Check sheet for the modelled part. Datum: model origin and axes. Units: mm. A direction names the side the tool comes from. Give positions to 0.01 mm unless a question says otherwise; leave off trailing zeros. Order: outer loops, then holes, each group sorted by start corner. A loop starts at its lowest first (then second) coordinate and runs counter-clockwise, first axis right, second up.
```python
from build123d import *

# Parameters (mm, degrees)
SKETCH1_W                = 30
SKETCH1_H                = 115
BOSS_EXTRUDE1_DEPTH      = 6.5
BOSS_EXTRUDE2_DEPTH      = 21.025
BOSS_EXTRUDE2_DEPTH_BACK = 21.025
SKETCH2_R                = 1.75
BOSS_EXTRUDE3_DEPTH      = 1.25
BOSS_EXTRUDE4_DEPTH      = 1.5
CUT_EXTRUDE1_DEPTH       = 176.585884356
CUT_EXTRUDE1_DEPTH_BACK  = 176.585884356
SKETCH5_W                = 15
SKETCH5_H                = 3.5
SKETCH5_W_2              = 3.5
CUT_EXTRUDE3_DEPTH       = 179.511058418
SPLIT1_SURFACE_1_1_BACK  = 238.381
SPLIT1_SURFACE_1_1_DEPTH = 476.762
SPLIT1_SURFACE_1_2_BACK  = 238.381
SPLIT1_SURFACE_1_2_DEPTH = 476.762
SPLIT1_SURFACE_2_3_BACK  = 238.381
SPLIT1_SURFACE_2_3_DEPTH = 476.762
SPLIT1_SURFACE_2_4_BACK  = 238.381
SPLIT1_SURFACE_2_4_DEPTH = 476.762
BOSS_EXTRUDE10_DEPTH     = 3.5
BOSS_EXTRUDE11_START     = -6.08688
BOSS_EXTRUDE11_DEPTH     = 3.91312
CUT_EXTRUDE4_DEPTH       = 177.703991537
CUT_EXTRUDE4_DEPTH_BACK  = 177.703991537


with BuildPart() as part:
    # Sketch1 → Boss-Extrude1 (new body)
    with BuildSketch(Plane(origin=(0, 0, 0), x_dir=(0, 0, 1), z_dir=(0, -1, 0))):
        Rectangle(SKETCH1_W, SKETCH1_H)
    extrude(amount=-BOSS_EXTRUDE1_DEPTH)

    # Sketch2 → Boss-Extrude2 (add, two sides: drawn at the far end of the back side and taken through both)
    with BuildSketch(Plane.XY.offset(-BOSS_EXTRUDE2_DEPTH_BACK)):
        with Locations(Location((-53.75, 3.25, 0), (0, 0, 180))):
            Circle(SKETCH2_R)
    extrude(amount=BOSS_EXTRUDE2_DEPTH + BOSS_EXTRUDE2_DEPTH_BACK)

    # Sketch4 → Boss-Extrude3 (add)
    with BuildSketch(Plane.ZY.offset(57.5)):
        Polygon((-1.044718626, 6.5), (-5.287359313, 6.5), (0, 1.212640687), (5.287359313, 6.5), (1.044718626, 6.5), (0, 5.455281374), align=None)
        Polygon((7.037359313, 12.492640687), (1.044718626, 6.5), (5.287359313, 6.5), (9.158679656, 10.371320344), align=None)
        Polygon((9.524051427, 14.964876926), (7.037359313, 12.492640687), (9.158679656, 10.371320344), (11.639169892, 12.837390757), align=None)
        Polygon((4.916038969, 14.613961031), (7.037359313, 12.492640687), (9.524051427, 14.964876926), (7.401708122, 17.099630183), align=None)
        Polygon((11.639169892, 12.837390757), (9.158679656, 10.371320344), (11.28, 8.25), (13.747117437, 10.717117437), align=None)
        Polygon((-7.037359313, 12.492640687), (-9.158679656, 10.371320344), (-5.287359313, 6.5), (-1.044718626, 6.5), align=None)
        Polygon((-11.28, 8.25), (-9.158679656, 10.371320344), (-11.639169892, 12.837390757), (-13.747117437, 10.717117437), align=None)
        Polygon((-11.639169892, 12.837390757), (-9.158679656, 10.371320344), (-7.037359313, 12.492640687), (-9.524051427, 14.964876926), align=None)
        Polygon((-9.524051427, 14.964876926), (-7.037359313, 12.492640687), (-4.916038969, 14.613961031), (-7.401708122, 17.099630183), align=None)
    extrude(amount=-BOSS_EXTRUDE3_DEPTH)

    # Sketch4<3> → Boss-Extrude4 (add)
    with BuildSketch(Plane.ZY.offset(57.5)):
        Polygon((-11.28, 8.25), (-9.158679656, 10.371320344), (-11.639169892, 12.837390757), (-13.747117437, 10.717117437), align=None)
        Polygon((-9.524051427, 14.964876926), (-7.037359313, 12.492640687), (-4.916038969, 14.613961031), (-7.401708122, 17.099630183), align=None)
        Polygon((4.916038969, 14.613961031), (7.037359313, 12.492640687), (9.524051427, 14.964876926), (7.401708122, 17.099630183), align=None)
        Polygon((11.639169892, 12.837390757), (9.158679656, 10.371320344), (11.28, 8.25), (13.747117437, 10.717117437), align=None)
    extrude(amount=BOSS_EXTRUDE4_DEPTH)

    # Mirror1: part across plane


with BuildPart() as part_1:
    add(part.part)
    add(part.part.mirror(Plane(origin=(57.5, 0, 0), x_dir=(0, 0, 1), z_dir=(1, 0, 0))))

    # Sketch6 → Cut-Extrude1 (cut, two sides: drawn at the far end of the back side and taken through both)
    with BuildSketch(Plane(origin=(0, 6.5, 0), x_dir=(1, 0, 0), z_dir=(0, 1, 0)).offset(-CUT_EXTRUDE1_DEPTH_BACK)):
        Polygon((162.5, 15), (-47.5, 15), (-37.5, -5), (-17.5, 5), (2.5, -5), (22.5, 7.5), (27.5, 2.5), (87.5, 2.5), (92.5, 7.5), (112.5, -5), (132.5, 5), (152.5, -5), align=None)
        Polygon((87.5, -5), (27.5, -5), (22.5, -10), (-37.5, -10), (-42.5, -15), (157.5, -15), (152.5, -10), (92.5, -10), align=None)
        Polygon((-2.326237921, -6.5), (-32.673762079, -6.5), (-17.5, 1.086881039), align=None)
        Polygon((25.025126266, -2.525126266), (21.050252532, -6.5), (6.703786792, -6.5), (21.993919555, 3.056332977), (25.025126266, 0.025126266), (26.300252532, -1.25), align=None)
        Polygon((93.949747468, -6.5), (108.296213208, -6.5), (93.006080445, 3.056332977), (89.974873734, 0.025126266), (88.699747468, -1.25), (89.974873734, -2.525126266), align=None)
        Polygon((132.5, 1.086881039), (117.326237921, -6.5), (147.673762079, -6.5), align=None)
    extrude(amount=CUT_EXTRUDE1_DEPTH + CUT_EXTRUDE1_DEPTH_BACK, mode=Mode.SUBTRACT)

    # Sketch5 → Cut-Extrude3 (cut, through all)
    with BuildSketch(Plane.XY.offset(-15)):
        with Locations((57.5, 6.5)):
            Rectangle(SKETCH5_W, SKETCH5_H)
        with Locations((40, 3.25)):
            Rectangle(SKETCH5_W_2, SKETCH5_H)
        with Locations((75, 3.25)):
            Rectangle(SKETCH5_W_2, SKETCH5_H)
        with Locations((57.5, 0)):
            Rectangle(SKETCH5_W, SKETCH5_H)
    extrude(amount=CUT_EXTRUDE3_DEPTH, mode=Mode.SUBTRACT)


with BuildPart() as body_2:
    # Split1: the piece behind the surface
    add(part_1.part)
    # Split1 surface 1: a surface, the sketch's curves swept straight by 476.762 mm
    with BuildLine(Plane(origin=(0, 0, 0), x_dir=(1, 0, 0), z_dir=(0, 1, 0)).offset(-SPLIT1_SURFACE_1_1_BACK), mode=Mode.PRIVATE) as split1_surface_1_1_path:
        Line((-27.5, 9.688914823), (-27.5, -15.311085177))
    split1_surface_1_1 = Shell.extrude(split1_surface_1_1_path.wire(), (0 * SPLIT1_SURFACE_1_1_DEPTH, 1 * SPLIT1_SURFACE_1_1_DEPTH, 0 * SPLIT1_SURFACE_1_1_DEPTH))
    split(bisect_by=split1_surface_1_1, keep=Keep.BOTTOM)


with BuildPart() as part_2:
    add(part_1.part)

    # Split1: split by a surface, the side it looks to stays
    # Split1 surface 1: a surface, the sketch's curves swept straight by 476.762 mm
    with BuildLine(Plane(origin=(0, 0, 0), x_dir=(1, 0, 0), z_dir=(0, 1, 0)).offset(-SPLIT1_SURFACE_1_2_BACK), mode=Mode.PRIVATE) as split1_surface_1_2_path:
        Line((-27.5, 9.688914823), (-27.5, -15.311085177))
    split1_surface_1_2 = Shell.extrude(split1_surface_1_2_path.wire(), (0 * SPLIT1_SURFACE_1_2_DEPTH, 1 * SPLIT1_SURFACE_1_2_DEPTH, 0 * SPLIT1_SURFACE_1_2_DEPTH))
    split(bisect_by=split1_surface_1_2, keep=Keep.TOP)


with BuildPart() as body_3:
    # Split1 2: the piece behind the surface
    add(part_2.part)
    # Split1 surface 2: a surface, the sketch's curves swept straight by 476.762 mm
    with BuildLine(Plane(origin=(0, 0, 0), x_dir=(1, 0, 0), z_dir=(0, 1, 0)).offset(-SPLIT1_SURFACE_2_3_BACK), mode=Mode.PRIVATE) as split1_surface_2_3_path:
        Line((142.5, 6.689515731), (142.5, -18.310484269))
    split1_surface_2_3 = Shell.extrude(split1_surface_2_3_path.wire(), (0 * SPLIT1_SURFACE_2_3_DEPTH, 1 * SPLIT1_SURFACE_2_3_DEPTH, 0 * SPLIT1_SURFACE_2_3_DEPTH))
    split(bisect_by=split1_surface_2_3, keep=Keep.BOTTOM)


with BuildPart() as part_3:
    add(part_2.part)

    # Split1 2: split by a surface, the side it looks to stays
    # Split1 surface 2: a surface, the sketch's curves swept straight by 476.762 mm
    with BuildLine(Plane(origin=(0, 0, 0), x_dir=(1, 0, 0), z_dir=(0, 1, 0)).offset(-SPLIT1_SURFACE_2_4_BACK), mode=Mode.PRIVATE) as split1_surface_2_4_path:
        Line((142.5, 6.689515731), (142.5, -18.310484269))
    split1_surface_2_4 = Shell.extrude(split1_surface_2_4_path.wire(), (0 * SPLIT1_SURFACE_2_4_DEPTH, 1 * SPLIT1_SURFACE_2_4_DEPTH, 0 * SPLIT1_SURFACE_2_4_DEPTH))
    split(bisect_by=split1_surface_2_4, keep=Keep.TOP)

    add(body_2.part)  # Boss-Extrude10 merges body 2


with BuildPart() as body_3_1:
    # Body-Move/Copy1: moved
    add(body_3.part.moved(Location((0, -22.5, 0))))


with BuildPart() as part_4:
    add(part_3.part)

    add(body_3_1.part)  # Boss-Extrude10 merges body 3
    # Sketch9 → Boss-Extrude10 (add)
    with BuildSketch(Plane.XY.offset(10)):
        Polygon((-27.5, -22.5), (-32.674762701, 0), (-27.5, 6.5), (-22.325237299, -16), align=None)
        Polygon((142.5, -22.5), (137.325237299, -16), (142.5, 6.5), (147.674762701, 0), align=None)
    extrude(amount=-BOSS_EXTRUDE10_DEPTH)

    # Sketch9<3> → Boss-Extrude11 (add)
    with BuildSketch(Plane.XY.offset(10).offset(BOSS_EXTRUDE11_START)):
        Polygon((-27.5, -22.5), (-32.674762701, 0), (-27.5, 6.5), (-22.325237299, -16), align=None)
        Polygon((142.5, -22.5), (137.325237299, -16), (142.5, 6.5), (147.674762701, 0), align=None)
    extrude(amount=-BOSS_EXTRUDE11_DEPTH)

    # Sketch11 → Cut-Extrude4 (cut, two sides: drawn at the far end of the back side and taken through both)
    with BuildSketch(Plane(origin=(0, 0, 0), x_dir=(1, 0, 0), z_dir=(0, 1, 0)).offset(-CUT_EXTRUDE4_DEPTH_BACK)):
        Polygon((-37.5, -5), (-17.5, 5), (-19.736067977, 9.472135955), (-39.736067977, -0.527864045), align=None)
        Polygon((-17.5, 1.086881039), (-32.673762079, -6.5), (-2.326237921, -6.5), align=None)
        Polygon((117.326237921, -6.5), (132.5, 1.086881039), (147.673762079, -6.5), align=None)
        Polygon((154.736067977, -0.527864045), (152.5, -5), (132.5, 5), (134.736067977, 9.472135955), align=None)
    extrude(amount=CUT_EXTRUDE4_DEPTH + CUT_EXTRUDE4_DEPTH_BACK, mode=Mode.SUBTRACT)


solid = part_4.part
```
(1) Sectioned sample at A-A (y = -9.5). Enter the section's corners in (x, z).
(2) Sectioned sample at C-C (x = 135). Enter the section's corners in (y, z).
(3) Tool access check on faces 1 (the face through (23.64, -19.3, 3.91)), 2 (the face through (-40, 3.2, 12.5)), 3 (the face through (-59, 11, 11)), 4 (the face through (-27.64, -8.2, 0.07)). Record the directions out of +Z, -Z, +X, -X, +Y, -Y that give a thin tool (end or side, any length) a straight path to the whole face; none if there is none.
(4) Go/stop test with flat-tipped pins: P1, Ø8, axis at x = 9, z = 15, coming from the -Y side; P2, Ø8, axis at x = 118.5, y = -13.5, coming from the +Z side; P3, Ø5, axis at y = -8.5, z = -1, coming from the -X side; P4, Ø14.5, axis at x = 129.5, y = -15, coming from the -Z side. Record where each tip stops, or that it passes through.
(5) Release check for a two-part mould opening along Z. For faces 5 (the face through (174, 15, -7)), 6 (the face through (90, -19.3, 7.5)), 7 (the face through (171.884, 9.454, -3.999)), 8 (the face through (24.18, -19.3, -0.87)) record: released by +Z, released by -Z, zero draft, split by the parting line, or undercut.
(6) Sectioned sample at B-B (z = 18). Enter the section's corners in (x, y).
(7) Thickness scan on L1, parallel to Y at x = 108.5, z = 8; L2, parallel to Y at x = -48, z = -9.5; L3, parallel to Z at x = 56, y = -20. Record the ranges inside material, lowest first.
Values follow:
1. outline: (-30.49, 1.49) - (-27.5, 0) - (-23.82, 0) - (-23.82, 2.07) - (-27.5, 3.91) - (-30.49, 3.91) - close; (-30.49, 6.5) - (-23.82, 6.5) - (-23.82, 10) - (-30.49, 10) - close; (138.82, 0) - (142.5, 0) - (145.49, 1.49) - (145.49, 3.91) - (142.5, 3.91) - (138.82, 2.07) - close; (138.82, 6.5) - (145.49, 6.5) - (145.49, 10) - (138.82, 10) - close
2. outline: (-22.5, -3.75) - (-16, -3.75) - (-16, 0.16) - (-22.5, 0.16) - close; (-22.5, 6.5) - (-16, 6.5) - (-16, 10) - (-22.5, 10) - close
3. face 1: +Y, -Y
3. face 2: +Z, +Y, -Y
3. face 3: +Z, -Z, -X, +Y, -Y
3. face 4: -Z, +Y, -Y
4. P1: passes through
4. P2: stops at z = 10
4. P3: stops at x = -30.5
4. P4: stops at z = -5
5. face 5: zero draft
5. face 6: released by +Z
5. face 7: undercut
5. face 8: undercut
6. outline: circle Ø3.5 at (-53.75, 3.25); circle Ø3.5 at (168.75, 3.25)
7. L1: y = -22.5 to -16
7. L2: y = 0 to 6.5
7. L3: z = -2.5 to 5
